Input: part model. Units: mm. Frame: model coordinates. A direction names the side the tool comes from. Coordinates: 2 decimals unless noted, no trailing zeros. Loops run counter-clockwise (first coordinate to the right, second up) from the corner with the lowest first, then second, coordinate; pieces in that order, holes last. Notation, with made-up numbers: M -3.5,3 L 28.5,3 A20 ccw 28.5,13 Z; hole C -16.75,83 d1. An arc over 180 degrees is marked long. Use a Markdown table: item, result. Add a question column.
1. Section A-A on x = 5.08. Output: boundary loops of the cut face in (y, z).
2. Set-up query: faces 4 (the flat face through (-4, 5, 6.909)), 5 (the cylindrical face through (-2.8, 22.64, 2.66)), 6 (the cylindrical face through (25.18, 4.96, 3.43)), 7 (the flat face through (17, 7.849, 0)). Return all of +Z, -Z, +X, -X, +Y, -Y with unobstructed straight access to the full face (end or side cutting, diameter ignored); none if empty.
3. Line query: L1, parallel to Z at x = 5.08, y = 1.15; L2, parallel to X at y = 1.3, z = 7.62; L3, parallel to Y at x = -5.5, z = -5. Output: solid intervals per line, ascending. Write a range as [from, to].
4. Pin query (flat end, axial travel): pin 1 (1.8 mm diameter, centred on x = -5.5, y = 6, fed in from -Z); pin 2 (5.5 mm diameter, centred on x = 11, z = 1, fed in from +Y); pin 3 (0.9 mm diameter, centred on x = 17.5, y = 6, fed in from -Z); pin 4 (5 mm diameter, centred on y = 16, z = 8, fed in from -X). Return the tip coordinate at first contact, or that it passes through.
5. Section C-C on x = 14.5. Output: boundary loops of the cut face in (y, z).
6. Section B-B on y = 11.5. Output: boundary loops of the cut face in (x, z).
7. Draft query along Y for faces 1 (the conical face through (-4.26, 28.88, 2.87)), 2 (the flat face through (-6, 15.672, 1)), 3 (the flat face through (31.623, 5, -6)). Return one class per face: +Y half, -Y half, draft (parallel to the pull), parting line (faces both ways), or undercut.
8. Section D-D on y = 20. Output: boundary loops of the cut face in (x, z).
```python
from build123d import *

# Parameters (mm, degrees)
SKETCH1_W           = 20.32
SKETCH1_H           = 20.447
BOSS_EXTRUDE1_DEPTH = 2.159
FILLET1_R           = 2.54
SKETCH2_W           = 6.9088
SKETCH2_H           = 15.113
BOSS_EXTRUDE2_DEPTH = 5.715
SKETCH3_W           = 11.9634
SKETCH3_H           = 13.8176
BOSS_EXTRUDE3_DEPTH = 6.1468
SKETCH4_R           = 4.8514
BOSS_EXTRUDE4_DEPTH = 0.254
SKETCH5_R           = 3.4036
BOSS_EXTRUDE5_DEPTH = 7.112
SKETCH6_R           = 1.651
BOSS_EXTRUDE6_DEPTH = 1.016
SKETCH7_R           = 2.9972
BOSS_EXTRUDE7_DEPTH = 12.319
CUT_EXTRUDE1_DEPTH  = 10.0838
SKETCH9_W           = 14.7828
SKETCH9_H           = 5.6642
BOSS_EXTRUDE8_DEPTH = 2.8448
SKETCH10_R          = 0.635
BOSS_EXTRUDE9_DEPTH = 12.7
SKETCH11_R          = 1.524
CUT_EXTRUDE2_DEPTH  = 12.7
CHAMFER1_SIZE       = 0.254


with BuildPart() as part:
    # Sketch1 → Boss-Extrude1 (new body)
    with BuildSketch(Plane(origin=(0, 0, 0), x_dir=(1, 0, 0), z_dir=(0, 1, 0))):
        Rectangle(SKETCH1_W, SKETCH1_H)
    extrude(amount=BOSS_EXTRUDE1_DEPTH)

    # Fillet1
    fillet1_edges = [part.edges().sort_by_distance(p)[0] for p in [
        (-10.16, 1.0795, -10.2235),
        (10.16, 1.0795, -10.2235),
        (10.16, 1.0795, 10.2235),
        (-10.16, 1.0795, 10.2235),
    ]]
    fillet(fillet1_edges, radius=FILLET1_R)

    # Sketch2 → Boss-Extrude2 (add)
    with BuildSketch(Plane(origin=(0, 2.159, 0), x_dir=(1, 0, 0), z_dir=(0, 1, 0))):
        with Locations((12.6238, 0)):
            Rectangle(SKETCH2_W, SKETCH2_H)
    extrude(amount=BOSS_EXTRUDE2_DEPTH)

    # Sketch3 → Boss-Extrude3 (add)
    with BuildSketch(Plane(origin=(0, 2.159, 0), x_dir=(1, 0, 0), z_dir=(0, 1, 0))):
        with Locations((-4.1783, 0)):
            Rectangle(SKETCH3_W, SKETCH3_H)
    extrude(amount=BOSS_EXTRUDE3_DEPTH)

    # Sketch4 → Boss-Extrude4 (add)
    with BuildSketch(Plane(origin=(0, 8.3058, 0), x_dir=(1, 0, 0), z_dir=(0, 1, 0))):
        with Locations((-4.1783, 0)):
            Circle(SKETCH4_R)
    extrude(amount=BOSS_EXTRUDE4_DEPTH)

    # Sketch5 → Boss-Extrude5 (add)
    with BuildSketch(Plane(origin=(0, 8.5598, 0), x_dir=(1, 0, 0), z_dir=(0, 1, 0))):
        with Locations((-4.1783, 0)):
            Circle(SKETCH5_R)
    extrude(amount=BOSS_EXTRUDE5_DEPTH)

    # Sketch6 → Boss-Extrude6 (add)
    with BuildSketch(Plane(origin=(0, 15.6718, 0), x_dir=(1, 0, 0), z_dir=(0, 1, 0))):
        with Locations((-4.1783, 0)):
            Circle(SKETCH6_R)
    extrude(amount=BOSS_EXTRUDE6_DEPTH)

    # Sketch7 → Boss-Extrude7 (add)
    with BuildSketch(Plane(origin=(0, 16.6878, 0), x_dir=(1, 0, 0), z_dir=(0, 1, 0))):
        with Locations((-4.1783, 0)):
            Circle(SKETCH7_R)
    extrude(amount=BOSS_EXTRUDE7_DEPTH)

    # Sketch8 → Cut-Extrude1 (cut)
    with BuildSketch(Plane(origin=(0, 29.0068, 0), x_dir=(1, 0, 0), z_dir=(0, 1, 0))):
        with BuildLine():
            Line((-6.78845126, 1.4732), (-1.56814874, 1.4732))
            ThreePointArc((-1.56814874, 1.4732), (-4.1783, 2.9972), (-6.78845126, 1.4732))
        make_face()
    extrude(amount=-CUT_EXTRUDE1_DEPTH, mode=Mode.SUBTRACT)

    # Sketch9 → Boss-Extrude8 (add)
    with BuildSketch(Plane(origin=(16.0782, 0, 0), x_dir=(0, 0, -1), z_dir=(1, 0, 0))):
        with Locations((0, 5.0165)):
            Rectangle(SKETCH9_W, SKETCH9_H)
    extrude(amount=BOSS_EXTRUDE8_DEPTH)

    # Sketch10 → Boss-Extrude9 (add)
    with BuildSketch(Plane(origin=(18.923, 0, 0), x_dir=(0, 0, -1), z_dir=(1, 0, 0))):
        with Locations((0, 4.935778059)):
            Circle(SKETCH10_R)
        with Locations((2.794, 4.935778059)):
            Circle(SKETCH10_R)
        with Locations((5.588, 4.935778059)):
            Circle(SKETCH10_R)
        with Locations((-2.794, 4.935778059)):
            Circle(SKETCH10_R)
        with Locations((-5.588, 4.935778059)):
            Circle(SKETCH10_R)
    extrude(amount=BOSS_EXTRUDE9_DEPTH)

    # Sketch11 → Cut-Extrude2 (cut)
    with BuildSketch(Plane(origin=(0, 2.159, 0), x_dir=(1, 0, 0), z_dir=(0, 1, 0))):
        with Locations((5.08, 7.62)):
            Circle(SKETCH11_R)
        with Locations((5.08, -7.62)):
            Circle(SKETCH11_R)
    extrude(amount=-CUT_EXTRUDE2_DEPTH, mode=Mode.SUBTRACT)

    # Chamfer1
    chamfer1_edges = [part.edges().sort_by_distance(p)[0] for p in [
        (-4.939897822, 29.0068, 2.898823313),
    ]]
    chamfer(chamfer1_edges, length=CHAMFER1_SIZE)


solid = part.part
```
Answers below:
| question | item | result |
|---|---|---|
| 1 | outline | M 0,-10.22 L 2.16,-10.22 L 2.16,-9.14 L 0,-9.14 Z; M 0,-6.1 L 2.16,-6.1 L 2.16,6.1 L 0,6.1 Z; M 0,9.14 L 2.16,9.14 L 2.16,10.22 L 0,10.22 Z |
| 2 | face 4 | +Z, -X, +Y |
| 2 | face 5 | +Y |
| 2 | face 6 | +X |
| 2 | face 7 | +Z, -Z, +X, +Y |
| 3 | L1 | z = [-10.22, -9.14], [-6.1, 6.1], [9.14, 10.22] |
| 3 | L2 | x = [-10.16, 3.56], [6.6, 10.16] |
| 3 | L3 | y = [0, 8.31] |
| 4 | pin 1 | stops at z = -6.91 |
| 4 | pin 2 | stops at y = 7.87 |
| 4 | pin 3 | stops at z = -7.39 |
| 4 | pin 4 | passes through |
| 5 | outline | M 2.16,-7.56 L 7.87,-7.56 L 7.87,7.56 L 2.16,7.56 Z |
| 6 | outline | C -4.18,0 d6.81 |
| 7 | face 1 | +Y half |
| 7 | face 2 | undercut |
| 7 | face 3 | draft |
| 8 | outline | M -6.79,-1.47 L -1.57,-1.47 A3 ccw long Z |
